```python
from build123d import *

# Parameters (mm, degrees)
EXTRUDE_1_DEPTH      = 2
CUT_EXTRUDE_1_REACH  = 306.145
SKETCH_3_R           = 13
SKETCH_3_R_2         = 1.65
SKETCH_6_OUTSIDE_W   = 723.656
SKETCH_6_OUTSIDE_H   = 223.656
SKETCH_6_OUTSIDE_W_2 = 773.893791272
SKETCH_6_OUTSIDE_H_2 = 70
CUT_EXTRUDE_4_DEPTH  = 10
SKETCH_7_W           = 40
SKETCH_7_H           = 125.252157634
SKETCH_7_H_2         = 116.31531122
CUT_EXTRUDE_5_DEPTH  = 10
FILLET_1_R           = 20
SKETCH_10_W          = 3
SKETCH_10_H          = 20
CUT_EXTRUDE_6_DEPTH  = 10


with BuildPart() as part:
    # 草图2 → 凸台-拉伸1 (new body)
    with BuildSketch(Plane.XY):
        with BuildLine():
            Line((-280, 50), (280, 50))
            ThreePointArc((280, 50), (294.142135624, 44.142135624), (300, 30))
            Line((300, 30), (300, -30))
            ThreePointArc((300, -30), (294.142135624, -44.142135624), (280, -50))
            Line((280, -50), (-280, -50))
            ThreePointArc((-280, -50), (-294.142135624, -44.142135624), (-300, -30))
            Line((-300, -30), (-300, 30))
            ThreePointArc((-300, 30), (-294.142135624, 44.142135624), (-280, 50))
        make_face()
    extrude(amount=EXTRUDE_1_DEPTH)

    # 草图3 → 切除-拉伸1 (cut, up to next)
    with BuildSketch(Plane.XY.offset(2), mode=Mode.PRIVATE) as cut_extrude_1_sk1:
        with Locations((-225, 0)):
            Circle(SKETCH_3_R)
    cut_extrude_1_tool1 = extrude(cut_extrude_1_sk1.sketch, amount=-CUT_EXTRUDE_1_REACH, mode=Mode.PRIVATE) & part.part
    # 草图3 → 切除-拉伸1 (cut, up to next)
    with BuildSketch(Plane.XY.offset(2), mode=Mode.PRIVATE) as cut_extrude_1_sk2:
        with Locations((225, 0)):
            Circle(SKETCH_3_R)
    cut_extrude_1_tool2 = extrude(cut_extrude_1_sk2.sketch, amount=-CUT_EXTRUDE_1_REACH, mode=Mode.PRIVATE) & part.part
    # 草图3 → 切除-拉伸1 (cut, up to next)
    with BuildSketch(Plane.XY.offset(2), mode=Mode.PRIVATE) as cut_extrude_1_sk3:
        with Locations((-242.5, 0)):
            Circle(SKETCH_3_R_2)
    cut_extrude_1_tool3 = extrude(cut_extrude_1_sk3.sketch, amount=-CUT_EXTRUDE_1_REACH, mode=Mode.PRIVATE) & part.part
    # 草图3 → 切除-拉伸1 (cut, up to next)
    with BuildSketch(Plane.XY.offset(2), mode=Mode.PRIVATE) as cut_extrude_1_sk4:
        with Locations((-207.5, 0)):
            Circle(SKETCH_3_R_2)
    cut_extrude_1_tool4 = extrude(cut_extrude_1_sk4.sketch, amount=-CUT_EXTRUDE_1_REACH, mode=Mode.PRIVATE) & part.part
    # 草图3 → 切除-拉伸1 (cut, up to next)
    with BuildSketch(Plane.XY.offset(2), mode=Mode.PRIVATE) as cut_extrude_1_sk5:
        with Locations((-225, 17.5)):
            Circle(SKETCH_3_R_2)
    cut_extrude_1_tool5 = extrude(cut_extrude_1_sk5.sketch, amount=-CUT_EXTRUDE_1_REACH, mode=Mode.PRIVATE) & part.part
    # 草图3 → 切除-拉伸1 (cut, up to next)
    with BuildSketch(Plane.XY.offset(2), mode=Mode.PRIVATE) as cut_extrude_1_sk6:
        with Locations((-225, -17.5)):
            Circle(SKETCH_3_R_2)
    cut_extrude_1_tool6 = extrude(cut_extrude_1_sk6.sketch, amount=-CUT_EXTRUDE_1_REACH, mode=Mode.PRIVATE) & part.part
    # 草图3 → 切除-拉伸1 (cut, up to next)
    with BuildSketch(Plane.XY.offset(2), mode=Mode.PRIVATE) as cut_extrude_1_sk7:
        with Locations((242.5, 0)):
            Circle(SKETCH_3_R_2)
    cut_extrude_1_tool7 = extrude(cut_extrude_1_sk7.sketch, amount=-CUT_EXTRUDE_1_REACH, mode=Mode.PRIVATE) & part.part
    # 草图3 → 切除-拉伸1 (cut, up to next)
    with BuildSketch(Plane.XY.offset(2), mode=Mode.PRIVATE) as cut_extrude_1_sk8:
        with Locations((225, 17.5)):
            Circle(SKETCH_3_R_2)
    cut_extrude_1_tool8 = extrude(cut_extrude_1_sk8.sketch, amount=-CUT_EXTRUDE_1_REACH, mode=Mode.PRIVATE) & part.part
    # 草图3 → 切除-拉伸1 (cut, up to next)
    with BuildSketch(Plane.XY.offset(2), mode=Mode.PRIVATE) as cut_extrude_1_sk9:
        with Locations((207.5, 0)):
            Circle(SKETCH_3_R_2)
    cut_extrude_1_tool9 = extrude(cut_extrude_1_sk9.sketch, amount=-CUT_EXTRUDE_1_REACH, mode=Mode.PRIVATE) & part.part
    # 草图3 → 切除-拉伸1 (cut, up to next)
    with BuildSketch(Plane.XY.offset(2), mode=Mode.PRIVATE) as cut_extrude_1_sk10:
        with Locations((225, -17.5)):
            Circle(SKETCH_3_R_2)
    cut_extrude_1_tool10 = extrude(cut_extrude_1_sk10.sketch, amount=-CUT_EXTRUDE_1_REACH, mode=Mode.PRIVATE) & part.part
    add(cut_extrude_1_tool1.solids().sort_by_distance((-225, 0, 2))[0], mode=Mode.SUBTRACT)
    add(cut_extrude_1_tool2.solids().sort_by_distance((225, 0, 2))[0], mode=Mode.SUBTRACT)
    add(cut_extrude_1_tool3.solids().sort_by_distance((-242.5, 0, 2))[0], mode=Mode.SUBTRACT)
    add(cut_extrude_1_tool4.solids().sort_by_distance((-207.5, 0, 2))[0], mode=Mode.SUBTRACT)
    add(cut_extrude_1_tool5.solids().sort_by_distance((-225, 17.5, 2))[0], mode=Mode.SUBTRACT)
    add(cut_extrude_1_tool6.solids().sort_by_distance((-225, -17.5, 2))[0], mode=Mode.SUBTRACT)
    add(cut_extrude_1_tool7.solids().sort_by_distance((242.5, 0, 2))[0], mode=Mode.SUBTRACT)
    add(cut_extrude_1_tool8.solids().sort_by_distance((225, 17.5, 2))[0], mode=Mode.SUBTRACT)
    add(cut_extrude_1_tool9.solids().sort_by_distance((207.5, 0, 2))[0], mode=Mode.SUBTRACT)
    add(cut_extrude_1_tool10.solids().sort_by_distance((225, -17.5, 2))[0], mode=Mode.SUBTRACT)

    # 草图6 outside → 切除-拉伸4 (cut)
    with BuildSketch(Plane.XY.offset(2)):
        Rectangle(SKETCH_6_OUTSIDE_W, SKETCH_6_OUTSIDE_H)
        Rectangle(SKETCH_6_OUTSIDE_W_2, SKETCH_6_OUTSIDE_H_2, mode=Mode.SUBTRACT)
    extrude(amount=-CUT_EXTRUDE_4_DEPTH, mode=Mode.SUBTRACT)

    # 草图7 → 切除-拉伸5 (cut)
    with BuildSketch(Plane.XY.offset(2)):
        with Locations((-300, 0)):
            Rectangle(SKETCH_7_W, SKETCH_7_H)
        with Locations((300, 0)):
            Rectangle(SKETCH_7_W, SKETCH_7_H_2)
    extrude(amount=-CUT_EXTRUDE_5_DEPTH, mode=Mode.SUBTRACT)

    # 圆角1
    fillet_1_edges = [part.edges().sort_by_distance(p)[0] for p in [
        (-280, 35, 1),
        (-280, -35, 1),
        (280, 35, 1),
        (280, -35, 1),
    ]]
    fillet(fillet_1_edges, radius=FILLET_1_R)

    # 草图10 → 切除-拉伸6 (cut)
    with BuildSketch(Plane.XY.offset(2)):
        with Locations((-75, 0)):
            Rectangle(SKETCH_10_W, SKETCH_10_H)
        with Locations((75, 0)):
            Rectangle(SKETCH_10_W, SKETCH_10_H)
    extrude(amount=-CUT_EXTRUDE_6_DEPTH, mode=Mode.SUBTRACT)


solid = part.part
```
Geometry check sheet. Reference: the model listing, model coordinates, mm. Give positions to 0.01 mm unless a question says otherwise; leave off trailing zeros. Write each loop counter-clockwise with the first axis right and the second up, starting at its lowest first coordinate (ties: lowest second). Pieces come first, ordered by that corner, then holes. Notation, with made-up numbers: (74, 67.5) - (115, 67.5) arc R16 cw to (115, 89.5) - close; hole circle Ø6 at (-2, -30). An arc over 180 degrees is marked (long way). Use a Markdown table: item, result.
Q1. Draft check along Y on faces 1 (the face through (-274.297, 28.986, 1.014)), 2 (the face through (4, 0, 2)), 3 (the face through (212.013, 0.572, 1.014)). Enter one of: pulls with the +Y half, pulls with the -Y half, needs draft (parallel to the pull), parting line crosses it, or undercut.
Computed:
| item | result |
|---|---|
| face 1 | pulls with the +Y half |
| face 2 | needs draft |
| face 3 | undercut |
Q2. Thickness scan on L1, parallel to Y at x = 225, z = 0.65; L2, parallel to X at y = 17, z = 1.15; L3, parallel to Y at x = -74.5, z = 1.65. Record the ranges inside material, lowest first. Write a range as [from, to].
Computed:
| item | result |
|---|---|
| L1 | y = [-35, -19.15], [-15.85, -13], [13, 15.85], [19.15, 35] |
| L2 | x = [-279.9, -226.57], [-223.43, 223.43], [226.57, 279.9] |
| L3 | y = [-35, -10], [10, 35] |
Q3. Section check B-B, the plane x = 231.5. Enter the section's corners in (y, z).
Computed:
| item | result |
|---|---|
| outline | (-35, 0) - (-11.26, 0) - (-11.26, 2) - (-35, 2) - close; (11.26, 0) - (35, 0) - (35, 2) - (11.26, 2) - close |
Q4. Section check A-A, the plane z = 0.9. Give the number of separate pieces and of enclosed holes in the cut face, then the cut area to 3 significant figures.
Computed:
| item | result |
|---|---|
| separate pieces | 1 |
| enclosed holes | 12 |
| area | 37,600 mm² |
